Build history of the part. All positions in model axes, mm. Coordinates: 2 decimals unless noted, no trailing zeros. Loops run counter-clockwise (first coordinate to the right, second up) from the corner with the lowest first, then second, coordinate; pieces in that order, holes last.
(1) Slice it at A-A (x = 15.24). Give the cut face in (y, z) (1 decimal), and give its area (3 significant figures).
(2) Wall check: L1, parallel to Y at x = 48.26, z = 1.2; L2, parallel to Y at x = 16, z = 1.8; L3, parallel to X at y = 44, z = 1.8. Give the ranges that are in metal, low to high.
(3) Two-plate mould, pull along Y, no slides. Class faces 1 (the face through (49.846, 6.407, 1.61)), 2 (the face through (31, 0, 2)), 3 (the face through (31, 26, 0)): pulls with the +Y half, pulls with the -Y half, needs draft (parallel to the pull), parting line crosses it, or undercut.
(4) Flat gauge pins, fed straight in: P1, Ø3, axis at x = 31, y = 37, coming from the -Z side; P2, Ø3, axis at x = 48.26, y = 6.477, coming from the -Z side. Where does each tip first touch, or does it go through?
from build123d import *

# Parameters (mm, degrees)
SKETCH1_W           = 63.5
SKETCH1_H           = 50.8
BOSS_EXTRUDE1_DEPTH = 3.175
FILLET1_R           = 2.54
SKETCH4_R           = 1.5875
CUT_EXTRUDE1_DEPTH  = 3.175


with BuildPart() as part:
    # Sketch1 → Boss-Extrude1 (new body)
    with BuildSketch(Plane.XY):
        with Locations((31.75, 25.4)):
            Rectangle(SKETCH1_W, SKETCH1_H)
    extrude(amount=BOSS_EXTRUDE1_DEPTH)

    # Fillet1
    fillet1_edges = [part.edges().sort_by_distance(p)[0] for p in [
        (0, 50.8, 1.5875),
        (63.5, 50.8, 1.5875),
        (63.5, 0, 1.5875),
        (0, 0, 1.5875),
    ]]
    fillet(fillet1_edges, radius=FILLET1_R)

    # Sketch4 → Cut-Extrude1 (cut)
    with BuildSketch(Plane.XY.offset(3.175)):
        with Locations(Location((15.24, 6.477, 0), (0, 0, 180))):
            Circle(SKETCH4_R)
        with Locations(Location((15.24, 44.323, 0), (0, 0, 180))):
            Circle(SKETCH4_R)
        with Locations(Location((48.26, 44.323, 0), (0, 0, 180))):
            Circle(SKETCH4_R)
        with Locations(Location((48.26, 6.477, 0), (0, 0, 180))):
            Circle(SKETCH4_R)
    extrude(amount=-CUT_EXTRUDE1_DEPTH, mode=Mode.SUBTRACT)


solid = part.part
Response values:
1. outline: (0, 0) - (4.9, 0) - (4.9, 3.2) - (0, 3.2) - close; (8.1, 0) - (42.7, 0) - (42.7, 3.2) - (8.1, 3.2) - close; (45.9, 0) - (50.8, 0) - (50.8, 3.2) - (45.9, 3.2) - close
1. area: 141 mm2
2. L1: y = 0 to 4.89, 8.06 to 42.74, 45.91 to 50.8
2. L2: y = 0 to 5.08, 7.87 to 42.93, 45.72 to 50.8
2. L3: x = 0 to 13.69, 16.79 to 46.71, 49.81 to 63.5
3. face 1: undercut
3. face 2: pulls with the -Y half
3. face 3: needs draft
4. P1: stops at z = 0
4. P2: passes through
